CAD build for the part. Positions are in the model's coordinates, mm. Give positions to 0.01 mm unless a question says otherwise; leave off trailing zeros. Write each loop counter-clockwise with the first axis right and the second up, starting at its lowest first coordinate (ties: lowest second). Pieces come first, ordered by that corner, then holes. Notation, with made-up numbers: (38, -25) - (80, -25) arc R22 cw to (80, -19) - close; hole circle Ø6 at (78.5, 18). An arc over 180 degrees is marked (long way). Put each result on its own line as item: value. Start each with the question number.
1. Cut at A-A on y = 24. List the corners of the cut face in (x, z), and give its area (3 significant figures).
2. Wall check: line 1 (X direction, y = 27.5, z = -0.1); line 2 (Y direction, x = 1.65, z = 0.5); line 3 (Y direction, x = 1.1, z = -0.2). Give the ranges that are in metal, low to high.
3. Drop a flat-ended pin along its axis: pin 1 (1 mm diameter, centred on y = 25.5, z = 1, fed in from +X). Give the stop position or say it passes through.
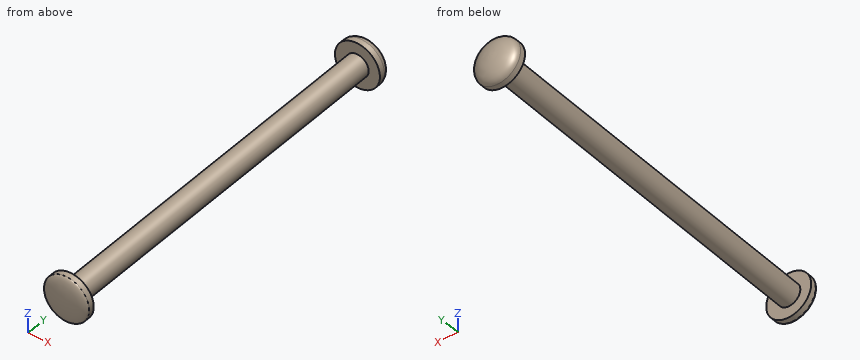
from build123d import *

# Parameters (mm, degrees)
SKETCH1_R                  = 1
MAIN_BODY_OF_SCREW_DEPTH   = 32
SKETCH2_R                  = 2
TOP_EXTRUDE_DEPTH          = 0.5
DOME_AT_TOP_FACE_RADIUS    = 2
DOME_AT_TOP_HEIGHT         = 1
SKETCH3_R                  = 2
BOTTOM_EXTRUDE_DEPTH       = 0.5
DOME_AT_BOTTOM_FACE_RADIUS = 2
DOME_AT_BOTTOM_HEIGHT      = 0.5


with BuildPart() as part:
    # Sketch1 → Main Body of Screw (new body)
    with BuildSketch(Plane(origin=(0, 0, 0), x_dir=(1, 0, 0), z_dir=(0, 1, 0))):
        with Locations(Location((0, 0, 0), (0, 0, 270))):
            Circle(SKETCH1_R)
    extrude(amount=MAIN_BODY_OF_SCREW_DEPTH)

    # Sketch2 → Top Extrude (add)
    with BuildSketch(Plane(origin=(0, 32, 0), x_dir=(1, 0, 0), z_dir=(0, 1, 0))):
        with Locations(Location((0, 0, 0), (0, 0, 270))):
            Circle(SKETCH2_R)
    extrude(amount=TOP_EXTRUDE_DEPTH)

    # Dome at Top: an elliptical dome of height H over a round flat face of radius A is half a spheroid: the quarter ellipse of half axes A and H revolved about the face's axis
    with BuildSketch(Plane((0, 32.5, 0), x_dir=(0, 0, -1), z_dir=(1, 0, 0)), mode=Mode.PRIVATE) as dome_at_top_quarter:
        Ellipse(DOME_AT_TOP_FACE_RADIUS, DOME_AT_TOP_HEIGHT)
        Rectangle(DOME_AT_TOP_FACE_RADIUS, DOME_AT_TOP_HEIGHT, align=(Align.MIN, Align.MIN), mode=Mode.INTERSECT)
    revolve(dome_at_top_quarter.sketch, axis=Axis((0, 32.5, 0), (0, 1, 0)))

    # Sketch3 → Bottom Extrude (add)
    with BuildSketch(Plane.XZ):
        with Locations(Location((0.033817747, 0, 0), (0, 0, 270))):
            Circle(SKETCH3_R)
    extrude(amount=BOTTOM_EXTRUDE_DEPTH)

    # Dome at Bottom: an elliptical dome of height H over a round flat face of radius A is half a spheroid: the quarter ellipse of half axes A and H revolved about the face's axis
    with BuildSketch(Plane((0.033817747, -0.5, 0), x_dir=(0, 0, 1), z_dir=(1, 0, 0)), mode=Mode.PRIVATE) as dome_at_bottom_quarter:
        Ellipse(DOME_AT_BOTTOM_FACE_RADIUS, DOME_AT_BOTTOM_HEIGHT)
        Rectangle(DOME_AT_BOTTOM_FACE_RADIUS, DOME_AT_BOTTOM_HEIGHT, align=(Align.MIN, Align.MIN), mode=Mode.INTERSECT)
    revolve(dome_at_bottom_quarter.sketch, axis=Axis((0.033817747, -0.5, 0), (0, -1, 0)))


solid = part.part
Report:
1. outline: circle Ø2 at (0, 0)
1. area: 3.14 mm²
2. line 1: x = -0.99 to 0.99
2. line 2: y = -0.77 to 0, 32 to 33.01
2. line 3: y = -0.92 to 0, 32 to 33.33
3. pin 1: stops at x = 0.87
